from build123d import *

# Parameters (mm, degrees)
F0_W     = 30.9265870601
F0_H     = 1.5
F1_DEPTH = 20
F2_START = 2
F2_DEPTH = 7.3
F4_DEPTH = 40


with BuildPart() as f1:
    # F0 (on Top) → F1 (new body)
    with BuildSketch(Plane.XY):
        with Locations((15.46329353, -13.2838593498)):
            Rectangle(F0_W, F0_H)
        with BuildLine():
            ThreePointArc((-6.9821200219, -12.5338593498), (-3.5707142143, -13.6546294884), (0, -14.0338593498))
            Line((0, -14.0338593498), (0, -12.5338593498))
            Line((0, -12.5338593498), (-6.9821200219, -12.5338593498))
        make_face()
    extrude(amount=F1_DEPTH)



with BuildPart() as f1b:
    # F0 (on Top) → F1, piece 2 (new body)
    with BuildSketch(Plane.XY):
        with Locations((15.46329353, -6.7838593498)):
            Rectangle(F0_W, F0_H)
        with BuildLine():
            Line((-13.3697419571, -7.5338593498), (0, -7.5338593498))
            Line((0, -7.5338593498), (0, -6.0338593498))
            Line((0, -6.0338593498), (-14.4222051019, -6.0338593498))
            ThreePointArc((-14.4222051019, -6.0338593498), (-13.9161984871, -6.7980500314), (-13.3697419571, -7.5338593498))
        make_face()
    extrude(amount=F1_DEPTH)


with BuildPart() as f1c:
    # F0 (on Top) → F1, piece 3 (new body)
    with BuildSketch(Plane.XY):
        with Locations((15.46329353, -0.2838593498)):
            Rectangle(F0_W, F0_H)
        with Locations((15.46329353, 6.2161406502)):
            Rectangle(F0_W, F0_H)
        with BuildLine():
            Line((-16.5227116419, -1.0338593498), (0, -1.0338593498))
            Line((0, -1.0338593498), (0, 0.4661406502))
            Line((0, 0.4661406502), (0, 5.4661406502))
            Line((0, 5.4661406502), (0, 6.9661406502))
            Line((0, 6.9661406502), (-16.5227116419, 6.9661406502))
            ThreePointArc((-16.5227116419, 6.9661406502), (-17, 2.9661406502), (-16.5227116419, -1.0338593498))
        make_face()
    extrude(amount=F1_DEPTH)


with BuildPart() as f1d:
    # F0 (on Top) → F1, piece 4 (new body)
    with BuildSketch(Plane.XY):
        with Locations((15.46329353, 12.7161406502)):
            Rectangle(F0_W, F0_H)
        with BuildLine():
            ThreePointArc((-13.3697419571, 13.4661406502), (-13.9161984871, 12.7303313319), (-14.4222051019, 11.9661406502))
            Line((-14.4222051019, 11.9661406502), (0, 11.9661406502))
            Line((0, 11.9661406502), (0, 13.4661406502))
            Line((0, 13.4661406502), (-13.3697419571, 13.4661406502))
        make_face()
    extrude(amount=F1_DEPTH)


with BuildPart() as f1e:
    # F0 (on Top) → F1, piece 5 (new body)
    with BuildSketch(Plane.XY):
        with Locations((15.46329353, 19.2161406502)):
            Rectangle(F0_W, F0_H)
        with BuildLine():
            ThreePointArc((0, 19.9661406502), (-3.5707142143, 19.5869107888), (-6.9821200219, 18.4661406502))
            Line((-6.9821200219, 18.4661406502), (0, 18.4661406502))
            Line((0, 18.4661406502), (0, 19.9661406502))
        make_face()
    extrude(amount=F1_DEPTH)


with BuildPart() as f1_1:
    add(f1.part)

    add(f1b.part)  # F2 merges F1b

    add(f1c.part)  # F2 merges F1c

    add(f1d.part)  # F2 merges F1d

    add(f1e.part)  # F2 merges F1e
    # F0 (on Top) → F2 (join)
    with BuildSketch(Plane.XY.offset(F2_START)):
        with BuildLine():
            Line((-6.9821200219, -12.5338593498), (0, -12.5338593498))
            Line((0, -12.5338593498), (0, -7.5338593498))
            Line((0, -7.5338593498), (-13.3697419571, -7.5338593498))
            ThreePointArc((-13.3697419571, -7.5338593498), (-10.4785290715, -10.4204357791), (-6.9821200219, -12.5338593498))
        make_face()
        with BuildLine():
            Line((-14.4222051019, -6.0338593498), (0, -6.0338593498))
            Line((0, -6.0338593498), (0, -1.0338593498))
            Line((0, -1.0338593498), (-16.5227116419, -1.0338593498))
            ThreePointArc((-16.5227116419, -1.0338593498), (-15.6731288538, -3.6181612817), (-14.4222051019, -6.0338593498))
        make_face()
        with BuildLine():
            Line((-16.5227116419, -1.0338593498), (0, -1.0338593498))
            Line((0, -1.0338593498), (0, 0.4661406502))
            Line((0, 0.4661406502), (0, 5.4661406502))
            Line((0, 5.4661406502), (0, 6.9661406502))
            Line((0, 6.9661406502), (-16.5227116419, 6.9661406502))
            ThreePointArc((-16.5227116419, 6.9661406502), (-17, 2.9661406502), (-16.5227116419, -1.0338593498))
        make_face()
        with BuildLine():
            ThreePointArc((-14.4222051019, 11.9661406502), (-15.6731288538, 9.5504425822), (-16.5227116419, 6.9661406502))
            Line((-16.5227116419, 6.9661406502), (0, 6.9661406502))
            Line((0, 6.9661406502), (0, 11.9661406502))
            Line((0, 11.9661406502), (-14.4222051019, 11.9661406502))
        make_face()
        with BuildLine():
            ThreePointArc((-6.9821200219, 18.4661406502), (-10.4785290715, 16.3527170795), (-13.3697419571, 13.4661406502))
            Line((-13.3697419571, 13.4661406502), (0, 13.4661406502))
            Line((0, 13.4661406502), (0, 18.4661406502))
            Line((0, 18.4661406502), (-6.9821200219, 18.4661406502))
        make_face()
    extrude(amount=F2_DEPTH)

    # F3 (on face) → F4 (intersect)
    with BuildSketch(Plane.XZ.offset(14.0338593498)):
        with BuildLine():
            Line((0, 6.1789047227), (-18.9112946391, 16.2631310523))
            ThreePointArc((-18.9112946391, 16.2631310523), (-12.4712318613, 4.6249463152), (0, 0))
            Line((0, 0), (0, 6.1789047227))
        make_face()
        Polygon((0, 6.1789047227), (0, 0), (30.9265870601, 0), (19.2144531757, 20), (24.9826789947, 3.5219495185), (4.9826789947, 3.5219495185), align=None)
    extrude(amount=-F4_DEPTH, mode=Mode.INTERSECT)


solid = f1_1.part
Read the model definition and answer for the solid it produces. Units are mm, in the model's axes. A direction names the side the tool comes from. Coordinates: 2 decimals unless noted, no trailing zeros. Write each loop counter-clockwise with the first axis right and the second up, starting at its lowest first coordinate (ties: lowest second). Pieces come first, ordered by that corner, then holes. Notation, with made-up numbers: (-6, 63.25) -> (46, 63.25) arc R19 ccw to (46, 88.25) -> close; hole circle Ø10 at (17.5, 33.25). An arc over 180 degrees is marked (long way). Return JSON: item names as keys, results as strings.
(1) The part is cut by section B-B on z = 17.5. Give the vertices of the cut face in (x, y).
Answers below:
{"outline": "(20.09, -14.03) -> (20.68, -14.03) -> (20.68, -12.53) -> (20.09, -12.53) -> close; (20.09, -7.53) -> (20.68, -7.53) -> (20.68, -6.03) -> (20.09, -6.03) -> close; (20.09, -1.03) -> (20.68, -1.03) -> (20.68, 0.47) -> (20.09, 0.47) -> close; (20.09, 5.47) -> (20.68, 5.47) -> (20.68, 6.97) -> (20.09, 6.97) -> close; (20.09, 11.97) -> (20.68, 11.97) -> (20.68, 13.47) -> (20.09, 13.47) -> close; (20.09, 18.47) -> (20.68, 18.47) -> (20.68, 19.97) -> (20.09, 19.97) -> close"}
(2) The part is cut by section A-A on x = 14. Give the vertices of the cut face in (y, z), then the cut area to 3 significant figures.
Answers below:
{"outline": "(-14.03, 0) -> (-12.53, 0) -> (-12.53, 3.52) -> (-14.03, 3.52) -> close; (-7.53, 0) -> (-6.03, 0) -> (-6.03, 3.52) -> (-7.53, 3.52) -> close; (-1.03, 0) -> (0.47, 0) -> (0.47, 3.52) -> (-1.03, 3.52) -> close; (5.47, 0) -> (6.97, 0) -> (6.97, 3.52) -> (5.47, 3.52) -> close; (11.97, 0) -> (13.47, 0) -> (13.47, 3.52) -> (11.97, 3.52) -> close; (18.47, 0) -> (19.97, 0) -> (19.97, 3.52) -> (18.47, 3.52) -> close", "area": "31.7 mm^2"}
(3) The part is cut by section C-C on z = 8.25. Give the vertices of the cut face in (x, y), then the cut area to 3 significant figures.
Answers below:
{"outline": "(-15.73, -3.47) arc R17 ccw to (-3.88, -13.58) -> (-3.88, 19.52) arc R17 ccw to (-15.73, 9.41) -> close; (23.33, -14.03) -> (26.1, -14.03) -> (26.1, -12.53) -> (23.33, -12.53) -> close; (23.33, -7.53) -> (26.1, -7.53) -> (26.1, -6.03) -> (23.33, -6.03) -> close; (23.33, -1.03) -> (26.1, -1.03) -> (26.1, 0.47) -> (23.33, 0.47) -> close; (23.33, 5.47) -> (26.1, 5.47) -> (26.1, 6.97) -> (23.33, 6.97) -> close; (23.33, 11.97) -> (26.1, 11.97) -> (26.1, 13.47) -> (23.33, 13.47) -> close; (23.33, 18.47) -> (26.1, 18.47) -> (26.1, 19.97) -> (23.33, 19.97) -> close", "area": "337 mm^2"}
(4) Which of the six approach directions +Z, -Z, +X, -X, +Y, -Y give full straight-line access (tool end or side, diameter ignored) to faces 4 (the flat face through (22.058, -13.294, 11.876)), 5 (the flat face through (-4, -3, 2)), 6 (the flat face through (17, 5.466, 3))?
Answers below:
{"face 4": "+Y, -Y", "face 5": "-Z, +X, -X", "face 6": "+Z, -Z, +X"}
(5) Consider line 1 along Y through (x, z) = (23, 2); line 2 along X through (y, z) = (13, 4.5); line 3 along Z through (x, y) = (-8, 17.5). Determine where each line is inside the solid, lowest interval first. Write a range as from..to.
Answers below:
{"line 1": "-14.03..-12.53, -7.53..-6.03, -1.03..0.47, 5.47..6.97, 11.97..13.47, 18.47..19.97", "line 2": "-12.32..3.15, 24.64..28.29", "line 3": "2..9.3"}
(6) The part is cut by section D-D on y = 6. Give the vertices of the cut face in (x, z).
Answers below:
{"outline": "(-16.73, 9.85) arc R19.13 ccw to (0, 0) -> (30.93, 0) -> (19.21, 20) -> (24.98, 3.52) -> (4.98, 3.52) -> (-16.73, 15.1) -> close"}
(7) For a pull along Z with two mould halves and no side action, classify faces 1 (the flat face through (22.058, -0.294, 11.876)), 2 (the flat face through (-11, 10, 9.3)), 3 (the flat face through (14, -1.034, 3)) as pulls with the +Z half, pulls with the -Z half, needs draft (parallel to the pull), parting line crosses it, or undercut.
Answers below:
{"face 1": "undercut", "face 2": "pulls with the +Z half", "face 3": "needs draft"}
(8) Each of these flat-tipped pins is pushed along its axis until it touches: P1, Ø3, axis at y = -7.5, z = 5, coming from the -X side; P2, Ø1.5, axis at y = -7, z = 17, coming from the -X side; P3, Ø1, axis at y = 2, z = 4.5, coming from the -X side; P4, Ø1.5, axis at y = 11, z = 14.5, coming from the +X side. Where does it stop, or does it pass through?
Answers below:
{"P1": "x = -14.07", "P2": "x = 20", "P3": "x = -12.89", "P4": "through"}
